The listing builds one solid part. Answer for the finished solid, in the listing's coordinates (mm). Face numbers are marked on the shaded views. A direction names the side the tool comes from. Coordinates: 2 decimals unless noted, no trailing zeros. Order: outer loops, then holes, each group sorted by start corner. A loop starts at its lowest first (then second) coordinate and runs counter-clockwise, first axis right, second up.
from build123d import *

# Parameters (mm, degrees)
SKETCH2_R           = 10
SKETCH2_R_2         = 1.5
BOSS_EXTRUDE1_DEPTH = 3
SKETCH3_R           = 4
BOSS_EXTRUDE2_DEPTH = 3
SKETCH4_R           = 1.5
CUT_EXTRUDE1_DEPTH  = 3


with BuildPart() as part:
    # Sketch2 → Boss-Extrude1 (new body)
    with BuildSketch(Plane(origin=(0, 0, 0), x_dir=(1, 0, 0), z_dir=(0, 1, 0))):
        Circle(SKETCH2_R)
        with Locations((0, -6.5)):
            Circle(SKETCH2_R_2, mode=Mode.SUBTRACT)
        with Locations((-6.5, 0)):
            Circle(SKETCH2_R_2, mode=Mode.SUBTRACT)
        with Locations((0, 6.5)):
            Circle(SKETCH2_R_2, mode=Mode.SUBTRACT)
        with Locations((6.5, 0)):
            Circle(SKETCH2_R_2, mode=Mode.SUBTRACT)
    extrude(amount=BOSS_EXTRUDE1_DEPTH)

    # Sketch3 → Boss-Extrude2 (add)
    with BuildSketch(Plane(origin=(0, 0, 0), x_dir=(-1, 0, 0), z_dir=(0, -1, 0))):
        Circle(SKETCH3_R)
    extrude(amount=BOSS_EXTRUDE2_DEPTH)

    # Sketch4 → Cut-Extrude1 (cut)
    with BuildSketch(Plane.XZ.offset(3)):
        Circle(SKETCH4_R)
    extrude(amount=-CUT_EXTRUDE1_DEPTH, mode=Mode.SUBTRACT)


solid = part.part
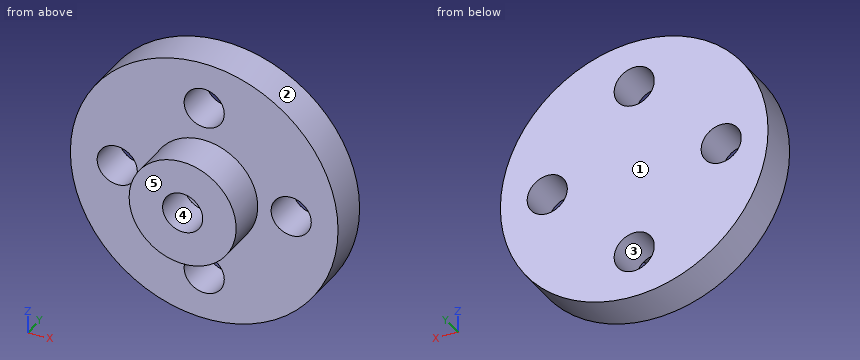
1) Section B-B (x = 6.5) is taken. Give the vertices of the cut face in (y, z), then the cut area to 3 significant figures.
2) Consider L1, parallel to X at y = 1.9, z = 0; L2, parallel to Z at x = 0, y = -1.65. Determine where each line is inside the solid, lowest interval first.
3) Section C-C (x = -0.25) is taken. Give the vertices of the cut face in (y, z), then the cut area to 3 significant figures.
4) A tool of negligible diameter and unlimited length cuts with its end or side. For the marked faces 4 and 5, from which of +Z, -Z, +X, -X, +Y, -Y can it reach the whole face along a straight path? Write none if from no direction.
5) Section D-D (y = 0.45) is taken. Give the vertices of the cut face in (x, z).
6) Determine the mould class of the marked faces 1, 2 and 3 for opening direction X: released by +X, released by -X, zero draft, split by the parting line, or undercut.
7) Section A-A (z = 0) is taken. Give the vertices of the cut face in (x, y).
8) Each of these flat-tipped pins is pushed along its axis until it touches: P1, Ø0.9, axis at x = -0.5, z = -0.5, coming from the -Y side; P2, Ø3, axis at x = 7, y = 2, coming from the +Z side; P3, Ø1, axis at y = 1, z = 5, coming from the +X side. Where does it stop, or does it pass through?
Filled sheet:
1. outline: (0, -7.6) - (3, -7.6) - (3, -1.5) - (0, -1.5) - close; (0, 1.5) - (3, 1.5) - (3, 7.6) - (0, 7.6) - close
1. area: 36.6 mm2
2. L1: x = -10 to -8, -5 to 5, 8 to 10
2. L2: z = -4 to -1.5, 1.5 to 4
3. outline: (-3, -3.99) - (0, -3.99) - (0, -5.02) - (3, -5.02) - (3, 5.02) - (0, 5.02) - (0, 3.99) - (-3, 3.99) - (-3, 1.48) - (0, 1.48) - (0, -1.48) - (-3, -1.48) - close; (0, -10) - (3, -10) - (3, -7.98) - (0, -7.98) - close; (0, 7.98) - (3, 7.98) - (3, 10) - (0, 10) - close
3. area: 57.3 mm2
4. face 4: -Y
4. face 5: +Z, -Z, +X, -X, -Y
5. outline: circle Ø20 at (0, 0); hole circle Ø3 at (-6.5, 0); hole circle Ø3 at (0, -6.5); hole circle Ø3 at (0, 6.5); hole circle Ø3 at (6.5, 0)
6. face 1: zero draft
6. face 2: split by the parting line
6. face 3: undercut
7. outline: (-10, 0) - (-8, 0) - (-8, 3) - (-10, 3) - close; (-5, 0) - (-4, 0) - (-4, -3) - (-1.5, -3) - (-1.5, 0) - (1.5, 0) - (1.5, -3) - (4, -3) - (4, 0) - (5, 0) - (5, 3) - (-5, 3) - close; (8, 0) - (10, 0) - (10, 3) - (8, 3) - close
8. P1: stops at y = 0
8. P2: stops at z = 8.35
8. P3: stops at x = 8.93
